```python
from build123d import *

# Parameters (mm, degrees)
SKETCH1_R               = 7.9375
SKETCH1_R_2             = 4.7625
BOSS_EXTRUDE1_DEPTH     = 60.579
SKETCH2_R               = 2.8575
CUT_EXTRUDE1_DEPTH      = 60.579
CUT_EXTRUDE1_DEPTH_BACK = 60.579
SKETCH3_R               = 1.5875
CUT_EXTRUDE2_DEPTH      = 60.579
CUT_EXTRUDE2_DEPTH_BACK = 60.579


with BuildPart() as part:
    # Sketch1 → Boss-Extrude1 (new body)
    with BuildSketch(Plane.XY):
        Circle(SKETCH1_R)
        Circle(SKETCH1_R_2, mode=Mode.SUBTRACT)
    extrude(amount=BOSS_EXTRUDE1_DEPTH)

    # Sketch2 → Cut-Extrude1 (cut, two sides)
    with BuildSketch(Plane(origin=(0, 0, 0), x_dir=(1, 0, 0), z_dir=(0, 1, 0))) as cut_extrude1_sk:
        with Locations((0, -14.605)):
            Circle(SKETCH2_R)
    extrude(amount=CUT_EXTRUDE1_DEPTH, mode=Mode.SUBTRACT)
    extrude(cut_extrude1_sk.sketch, amount=-CUT_EXTRUDE1_DEPTH_BACK, mode=Mode.SUBTRACT)

    # Sketch3 → Cut-Extrude2 (cut, two sides)
    with BuildSketch(Plane(origin=(0, 0, 0), x_dir=(1, 0, 0), z_dir=(0, 1, 0))) as cut_extrude2_sk:
        with Locations((0, -27.94)):
            Circle(SKETCH3_R)
    extrude(amount=CUT_EXTRUDE2_DEPTH, mode=Mode.SUBTRACT)
    extrude(cut_extrude2_sk.sketch, amount=-CUT_EXTRUDE2_DEPTH_BACK, mode=Mode.SUBTRACT)


solid = part.part
```
Source: CAD feature listing. Evaluate the final solid. Frame: model axes, mm. Coordinates: 2 decimals unless noted, no trailing zeros. Write each loop counter-clockwise with the first axis right and the second up, starting at its lowest first coordinate (ties: lowest second). Pieces come first, ordered by that corner, then holes. Notation, with made-up numbers: (38.25, 51.5) -> (53.25, 51.5) arc R17 ccw to (53.25, 62.5) -> close; hole circle Ø8 at (45, 50). An arc over 180 degrees is marked (long way). Return JSON: item names as keys, results as strings. Group by question number.
1) Section query D-D, the plane z = 9. Return loops of the section in (x, y) (1 decimal), plus the area to 3 significant figures.
2) Section query B-B, the plane y = 0. Return loops of the section in (x, z).
3) Mould query, pull axis X, two halves, no side actions, for faces 1 (the face through (0, -5, 60.579)), 2 (the face through (7.332, -3.04, 29.865)), 3 (the face through (2.64, 5.85, 15.7)). Classes: +X half, -X half, draft (parallel to the pull), parting line (faces both ways), or undercut.
4) Ray query, line 1 along Z through (x, y) = (0, -7); line 2 along X through (y, z) = (1.25, 25); line 3 along Y through (x, z) = (3.75, 29). Return the intervals inside material, ascending.
5) Section query A-A, the plane x = 0. Return loops of the section in (y, z).
6) Contact query for flat-ended pins moving along their axis: P1, Ø5, axis at x = 0, z = 27.94, coming from the +Y side; P2, Ø1.9, axis at x = 0, z = 27.94, coming from the -Y side; P3, Ø4, axis at y = -5.5, z = 24.5, coming from the -X side; P4, Ø3, axis at x = -6, z = 12, coming from the +Y side. Output: stop coordinate, or through.
From the geometry:
{
 "1": {"outline": "circle Ø15.9 at (0, 0); hole circle Ø9.5 at (0, 0)", "area": "127 mm²"},
 "2": {"outline": "(-7.94, 0) -> (-4.76, 0) -> (-4.76, 60.58) -> (-7.94, 60.58) -> close; (4.76, 0) -> (7.94, 0) -> (7.94, 60.58) -> (4.76, 60.58) -> close"},
 "3": {"face 1": "draft", "face 2": "parting line", "face 3": "undercut"},
 "4": {"line 1": "0 to 11.75, 17.46 to 26.35, 29.53 to 60.58", "line 2": "-7.84 to -4.6, 4.6 to 7.84", "line 3": "-7 to -2.94, 2.94 to 7"},
 "5": {"outline": "(-7.94, 0) -> (-4.76, 0) -> (-4.76, 11.75) -> (-7.94, 11.75) -> close; (-7.94, 17.46) -> (-4.76, 17.46) -> (-4.76, 26.35) -> (-7.94, 26.35) -> close; (-7.94, 29.53) -> (-4.76, 29.53) -> (-4.76, 60.58) -> (-7.94, 60.58) -> close; (4.76, 0) -> (7.94, 0) -> (7.94, 11.75) -> (4.76, 11.75) -> close; (4.76, 17.46) -> (7.94, 17.46) -> (7.94, 26.35) -> (4.76, 26.35) -> close; (4.76, 29.53) -> (7.94, 29.53) -> (7.94, 60.58) -> (4.76, 60.58) -> close"},
 "6": {"P1": "y = 7.94", "P2": "through", "P3": "x = -7.12", "P4": "y = 6.54"}
}
